```python
from build123d import *

# Parameters (mm, degrees)
F0_R     = 1.5
F1_DEPTH = 1.25


with BuildPart() as f1:
    # F0 (on Front) → F1 (new body, symmetric)
    with BuildSketch(Plane.XZ):
        Polygon((-6.936875, 37.129661), (-31.911666, 40.025616), (-23.51977, 3.25795), align=None)
        with Locations((-21.79202, 18.158109)):
            Circle(F0_R, mode=Mode.SUBTRACT)
        with Locations((-25.463581, 34.244427)):
            Circle(F0_R, mode=Mode.SUBTRACT)
        with Locations((-14.536794, 32.97741)):
            Circle(F0_R, mode=Mode.SUBTRACT)
    extrude(amount=F1_DEPTH, both=True)


solid = f1.part
```
CAD build for the part. Positions are in the model's coordinates, mm. Give positions to 0.01 mm unless a question says otherwise; leave off trailing zeros. Order: outer loops, then holes, each group sorted by start corner. A loop starts at its lowest first (then second) coordinate and runs counter-clockwise, first axis right, second up.
(1) Saw through at C-C, the plane y = -0.45. Give the cut face in (x, z).
(2) Drill centre lines: L1, parallel to Z at x = -20.75, y = -1; L2, parallel to Z at x = -14.5, y = -0.65; L3, parallel to Z at x = -18.25, y = -0.25. Where is each one in solid material? Low to high.
(3) Saw through at B-B, the plane z = 19. Give the cut face in (x, y), then the cut area to 3 significant figures.
(4) Saw through at A-A, the plane x = -25. Give the cut face in (y, z).
(5) Flat gauge pins, fed straight in: pin 1 (1.5 mm diameter, centred on y = 0.5, z = 16.5, fed in from -X); pin 2 (1 mm diameter, centred on y = 0.5, z = 8, fed in from -X); pin 3 (1.5 mm diameter, centred on x = -19, y = 0.5, fed in from -Z); pin 4 (2.5 mm diameter, centred on x = -25.46, z = 34.24, fed in from +Y). Where does each tip first touch, or does it go through?
(6) Saw through at D-D, the plane z = 13.5. Give the cut face in (x, y), then the cut area to 3 significant figures.
(7) Mould opens along X. For faces 1 (the cylindrical face through (-13.73, 0.02, 34.24)), 2 (the flat face through (-20, 1.25, 26)), 3 (the flat face through (-19.249, -0.018, 38.557)) say: released by +X, released by -X, zero draft, split by the parting line, or undercut.
Results found:
1. outline: (-31.91, 40.03) - (-23.52, 3.26) - (-6.94, 37.13) - close; hole circle Ø3 at (-25.46, 34.24); hole circle Ø3 at (-21.79, 18.16); hole circle Ø3 at (-14.54, 32.98)
2. L1: z = 8.92 to 17.08, 19.24 to 38.73
2. L2: z = 21.68 to 31.48, 34.48 to 38.01
2. L3: z = 14.02 to 38.44
3. outline: (-27.11, -1.25) - (-23.03, -1.25) - (-23.03, 1.25) - (-27.11, 1.25) - close; (-20.55, -1.25) - (-15.81, -1.25) - (-15.81, 1.25) - (-20.55, 1.25) - close
3. area: 22.0 mm2
4. outline: (-1.25, 9.74) - (1.25, 9.74) - (1.25, 32.82) - (-1.25, 32.82) - close; (-1.25, 35.67) - (1.25, 35.67) - (1.25, 39.22) - (-1.25, 39.22) - close
5. pin 1: stops at x = -26.71
5. pin 2: stops at x = -24.72
5. pin 3: stops at z = 10.96
5. pin 4: passes through
6. outline: (-25.86, -1.25) - (-18.51, -1.25) - (-18.51, 1.25) - (-25.86, 1.25) - close
6. area: 18.4 mm2
7. face 1: undercut
7. face 2: zero draft
7. face 3: released by +X
